For this review, take the finished solid that the model builds, in its own axes (mm). Face numbers are marked on the shaded views. A direction names the side the tool comes from. Round coordinates to 2 decimals unless told otherwise and drop trailing zeros. Loops run counter-clockwise (first coordinate to the right, second up) from the corner with the lowest first, then second, coordinate; pieces in that order, holes last.
Autodesk Inventor part; units mm, degrees
ref_plane "YZ Plane" through (0, 0, 0) normal (1, 0, 0) x (0, 1, 0)
ref_plane "XZ Plane" through (0, 0, 0) normal (0, 1, 0) x (-1, 0, 0)
ref_plane "XY Plane" through (0, 0, 0) normal (0, 0, 1) x (1, 0, 0)
sketch "Sketch1" plane through (0, 0, 0) normal (0, 0, 1) x (1, 0, 0)
  line L0 (-2, 0) -> (-2, -16)
  line L1 (-2, -16) -> (-4, -16)
  line L2 (-4, -16) -> (-4, -2)
  line L3 (-4, -2) -> (-12, -2)
  line L4 (-12, -2) -> (-12, 0)
  line L5 (-12, 0) -> (-2, 0)
  line L6 (-12, 0) -> (-2, 0)
  dimension "d38" = 2
  dimension "d39" = 14
  dimension "d40" = 8
  dimension "d41" = 2
extrude "Extrusion3" add sketch "Sketch1" along normal blind 15
sketch "Sketch2" plane through (-12, -2, 0) normal (0, -1, 0) x (1, 0, 0)
  circle A0 centre (4, 4.25) radius 1.5
  line L0 (0, 15) -> (8, 15)
  line L1 (0, 0) -> (0, 15)
  line L2 (0, 0) -> (8, 0)
  circle A1 centre (4, 10.75) radius 1.5
  dimension "d45" = 3
  dimension "d47" = 4
  dimension "d48" = 4.25
  dimension "d49" = 3
  dimension "d50" = 4
  dimension "d51" = 4.25
extrude "Extrusion4" cut sketch "Sketch2" against normal blind 10
sketch "Sketch3" plane through (-4, -16, 0) normal (-1, 0, 0) x (0, 0, 1)
  circle A0 centre (12, 5.4) radius 1.5
  circle A1 centre (3, 5.4) radius 1.5
  line L0 (0, 0) -> (15, 0)
  line L1 (15, 14) -> (15, 0)
  line L2 (0, 14) -> (0, 0)
  circle A2 centre (7.5, 10) radius 2
  dimension "d55" = 3
  dimension "d56" = 5.4
  dimension "d57" = 5.4
  dimension "d58" = 3
  dimension "d59" = 3
  dimension "d62" = 4
  dimension "d65" = 10
  dimension "d68" = 3
extrude "Extrusion5" cut sketch "Sketch3" against normal blind 10 contours A0 | A1
extrude "Extrusion6" cut sketch "Sketch3" against normal blind 10 contours A2
fillet "Fillet1" radius 2.5 1 edges at (-2, 0, 7.5)
fillet "Fillet2" radius 0.5 1 edges at (-4, -2, 7.5)
equation "\"d48\" = d51"
properties part number "Soporte de Final de Carrera - Eje Y" material "Aluminum 1100-H14"
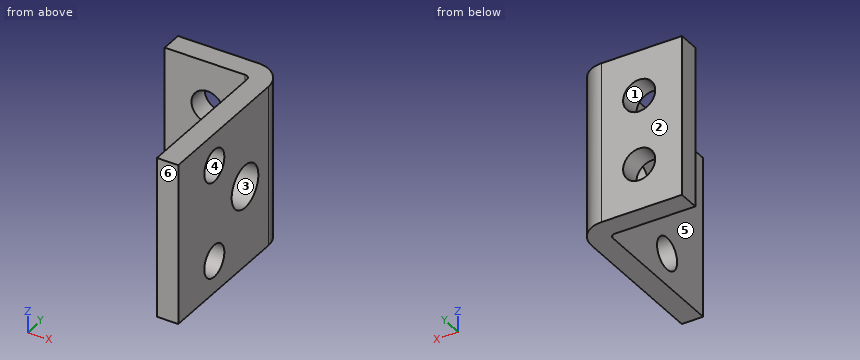
(1) Add section C-C (z = 10). Give the boundary of the cut face in (x, y), plus the area to 3 significant figures.
(2) Add section B-B (x = -7). Give the boundary of the cut face in (y, z), plus the area to 3 significant figures.
(3) For the marked faces 5 and 6, list the 3-axis set-ups (+Z, -Z, +X, -X, +Y, -Y) from which the entire face can be reached by the end or side of a thin tool; tool diameter is ignored.
(4) Insertion check: pin 1 Ø2 at (x, z) = (-9.5, 11) entering from -Y; pin 2 Ø1.8 at (x, z) = (-8, 4.25) entering from -Y. Each pin has a flat end and moves straight along its axis. Give the tip position at first contact, or say it passes through.
(5) Add section D-D (y = -6). Give the boundary of the cut face in (x, z).
(6) Add section A-A (y = -10.6). Give the boundary of the cut face in (x, z).
(7) The part is to be moulded in two halves that separate along Y. For the marked faces 1, 2, 3 and 4, say which applies: pulls with the +Y half, pulls with the -Y half, needs draft (parallel to the pull), parting line crosses it, or undercut.
(8) For L1, parallel to Z at x = -8, y = -1.15; L2, parallel to X at y = -7, z = 3.5; L3, parallel to Y at x = -8, z = 12.75, list the stretches that pass through material, from the lowest coordinate up.
Outcome:
1. outline: (-12, -2) - (-9.3, -2) - (-9.3, 0) - (-12, 0) - close; (-6.7, -2) - (-4.5, -2) arc R0.5 cw to (-4, -2.5) - (-4, -16) - (-2, -16) - (-2, -2.5) arc R2.5 ccw to (-4.5, 0) - (-6.7, 0) - close
1. area: 41.5 mm2
2. outline: (-2, 0) - (0, 0) - (0, 3.13) - (-2, 3.13) - close; (-2, 5.37) - (0, 5.37) - (0, 9.63) - (-2, 9.63) - close; (-2, 11.87) - (0, 11.87) - (0, 15) - (-2, 15) - close
2. area: 21.1 mm2
3. face 5: +Z, -Z, -X, -Y
3. face 6: +Z, -Z, +X, -X, -Y
4. pin 1: stops at y = -2
4. pin 2: passes through
5. outline: (-4, 0) - (-2, 0) - (-2, 5.5) - (-4, 5.5) - close; (-4, 9.5) - (-2, 9.5) - (-2, 15) - (-4, 15) - close
6. outline: (-4, 0) - (-2, 0) - (-2, 1.5) - (-4, 1.5) - close; (-4, 4.5) - (-2, 4.5) - (-2, 10.5) - (-4, 10.5) - close; (-4, 13.5) - (-2, 13.5) - (-2, 15) - (-4, 15) - close
7. face 1: needs draft
7. face 2: pulls with the +Y half
7. face 3: undercut
7. face 4: undercut
8. L1: z = 0 to 2.75, 5.75 to 9.25, 12.25 to 15
8. L2: x = -4 to -2
8. L3: y = -2 to 0
